```python
from build123d import *

# Parameters (mm, degrees)
SKETCH2_W           = 256
SKETCH2_H           = 186
BOSS_EXTRUDE1_DEPTH = 3
SKETCH3_R           = 1.6
CUT_EXTRUDE1_DEPTH  = 4
SKETCH4_R           = 2
SKETCH4_W           = 12.5
SKETCH4_H           = 11
CUT_EXTRUDE2_DEPTH  = 10
FILLET1_R           = 1
SKETCH5_R           = 4.5
CUT_EXTRUDE3_DEPTH  = 10
SKETCH7_R           = 1.5
CUT_EXTRUDE4_DEPTH  = 4
FILLET2_R           = 1


with BuildPart() as part:
    # Sketch2 → Boss-Extrude1 (new body)
    with BuildSketch(Plane.XY):
        with Locations((128, 93)):
            Rectangle(SKETCH2_W, SKETCH2_H)
    extrude(amount=BOSS_EXTRUDE1_DEPTH)

    # Sketch3 → Cut-Extrude1 (cut, through all)
    with BuildSketch(Plane.XY.offset(3)):
        with Locations((6, 176)):
            Circle(SKETCH3_R)
        with Locations((128, 180)):
            Circle(SKETCH3_R)
        with Locations((246, 180)):
            Circle(SKETCH3_R)
        with Locations((246, 6)):
            Circle(SKETCH3_R)
        with Locations((128, 6)):
            Circle(SKETCH3_R)
        with Locations((6, 10)):
            Circle(SKETCH3_R)
    extrude(amount=-CUT_EXTRUDE1_DEPTH, mode=Mode.SUBTRACT)

    # Sketch4 → Cut-Extrude2 (cut)
    with BuildSketch(Plane.XY.offset(3)):
        with Locations((35, 25.5)):
            Circle(SKETCH4_R)
        with Locations((63, 25.5)):
            Circle(SKETCH4_R)
        with Locations((49, 25.5)):
            Rectangle(SKETCH4_W, SKETCH4_H)
    extrude(amount=-CUT_EXTRUDE2_DEPTH, mode=Mode.SUBTRACT)

    # Fillet1
    fillet1_edges = [part.edges().sort_by_distance(p)[0] for p in [
        (42.75, 20, 1.5),
        (42.75, 31, 1.5),
        (55.25, 31, 1.5),
        (55.25, 20, 1.5),
    ]]
    fillet(fillet1_edges, radius=FILLET1_R)

    # Sketch5 → Cut-Extrude3 (cut)
    with BuildSketch(Plane.XY.offset(3)):
        with Locations((20, 35)):
            Circle(SKETCH5_R)
        with Locations((20, 20)):
            Circle(SKETCH5_R)
        with Locations((20, 50)):
            Circle(SKETCH5_R)
    extrude(amount=-CUT_EXTRUDE3_DEPTH, mode=Mode.SUBTRACT)

    # Sketch7 → Cut-Extrude4 (cut, through all)
    with BuildSketch(Plane(origin=(161.992525703, 0.203186411, 3), x_dir=(1, 0, 0), z_dir=(0, 0, 1))):
        with Locations((-140.992525703, 112.796813589)):
            Circle(SKETCH7_R)
        with Locations((-140.992525703, 79.796813589)):
            Circle(SKETCH7_R)
        Polygon((-146.992525703, 110.796813589), (-146.992525703, 81.796813589), (-134.992525703, 82.796813589), (-134.992525703, 109.796813589), align=None)
    extrude(amount=-CUT_EXTRUDE4_DEPTH, mode=Mode.SUBTRACT)

    # Fillet2
    fillet2_edges = [part.edges().sort_by_distance(p)[0] for p in [
        (15, 111, 1.5),
        (27, 110, 1.5),
        (27, 83, 1.5),
        (15, 82, 1.5),
    ]]
    fillet(fillet2_edges, radius=FILLET2_R)


solid = part.part
```
Can you work these out from the model? Positions are in its coordinate system, mm. Round coordinates to 2 decimals unless told otherwise and drop trailing zeros. Loops run counter-clockwise (first coordinate to the right, second up) from the corner with the lowest first, then second, coordinate; pieces in that order, holes last.
Item 1: Suppose I cut it at B-B, the plane y = 50. Write out the boundary of the cut face in (x, z), then the cut area to 3 significant figures.
Item 2: If we mould it in two halves opening along Y, with no side actions, what happens to faces 1 (the cylindrical face through (16.68, 23.04, 1.52)), 2 (the flat face through (126, 94, 3))? For each: +Y half, -Y half, draft (parallel to the pull), parting line (faces both ways), or undercut.
Item 3: Please list where these lines run through material, in increasing order: L1, parallel to Y at x = 246, z = 0.9; L2, parallel to X at y = 80, z = 1.9; L3, parallel to X at y = 97.5, z = 2.35.
Item 4: Suppose I cut it at A-A, the plane z = 0.85. State how many separate pieces and enclosed holes the cut face has, then the cut area to 3 significant figures.
Reported:
1. outline: (0, 0) - (15.5, 0) - (15.5, 3) - (0, 3) - close; (24.5, 0) - (256, 0) - (256, 3) - (24.5, 3) - close
1. area: 741 mm2
2. face 1: undercut
2. face 2: draft
3. L1: y = 0 to 4.4, 7.6 to 178.4, 181.6 to 186
3. L2: x = 0 to 19.5, 22.5 to 256
3. L3: x = 0 to 15, 27 to 256
4. separate pieces: 1
4. enclosed holes: 15
4. area: 46,900 mm2
